For this review, use the dimensioned drawing (mm, ordinates from the lowest corner) and the shaded views. A direction names the side the tool comes from. Round coordinates to 2 decimals unless told otherwise and drop trailing zeros. Loops run counter-clockwise (first coordinate to the right, second up) from the corner with the lowest first, then second, coordinate; pieces in that order, holes last. Notation, with made-up numbers: (24.25, 84.5) -> (52.25, 84.5) arc R38 cw to (52.25, 123.5) -> close; hole circle Ø4 at (51, 89). An arc over 180 degrees is marked (long way). Write each question's results on one line, items separated by ' | '.
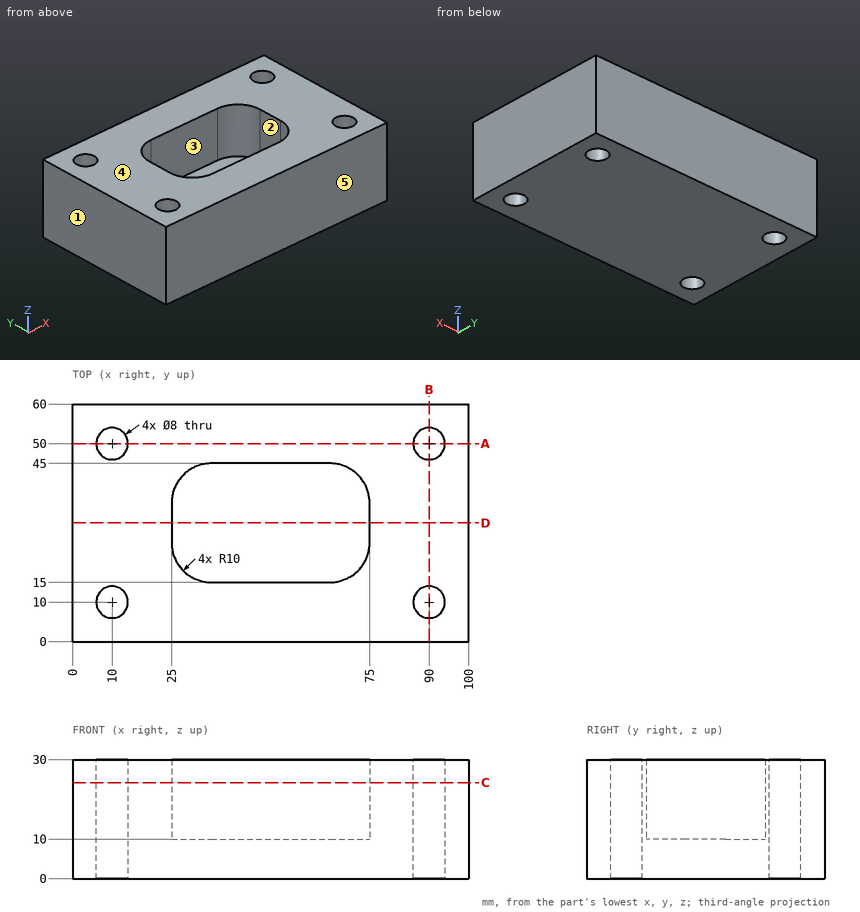
1. Draft analysis for pull direction Y (two halves, no side actions). For the marked faces 3, 4 and 5, state which applies: released by +Y, released by -Y, zero draft, split by the parting line, or undercut.
Values found:
face 3: undercut | face 4: zero draft | face 5: released by -Y
2. For pin 1 (5 mm diameter, centred on x = 10, y = 10, fed in from -Z); pin 2 (5 mm diameter, centred on x = 41, y = 22.5, fed in from +Z), all flat-tipped, find the tip position at first contact; note any pin that passes through.
Values found:
pin 1: passes through | pin 2: stops at z = 10
3. To check wall thickness, follow probe 1 along Y at (x, z) = (90, 19.25); probe 2 along Y at (x, z) = (57, 24); probe 3 along X at (y, z) = (50.5, 16.75). State the ranges of each line that lie inside material, in increasing order.
Values found:
probe 1: y = 0 to 6, 14 to 46, 54 to 60 | probe 2: y = 0 to 15, 45 to 60 | probe 3: x = 0 to 6.03, 13.97 to 86.03, 93.97 to 100
4. Consider section A-A (y = 50). State the section outline as (x, z) points.
Values found:
outline: (0, 0) -> (6, 0) -> (6, 30) -> (0, 30) -> close; (14, 0) -> (86, 0) -> (86, 30) -> (14, 30) -> close; (94, 0) -> (100, 0) -> (100, 30) -> (94, 30) -> close
5. Consider section D-D (y = 30). State the section outline as (x, z) points.
Values found:
outline: (0, 0) -> (100, 0) -> (100, 30) -> (75, 30) -> (75, 10) -> (25, 10) -> (25, 30) -> (0, 30) -> close
6. Consider section B-B (x = 90). State the section outline as (y, z) points, plus the area to 3 significant figures.
Values found:
outline: (0, 0) -> (6, 0) -> (6, 30) -> (0, 30) -> close; (14, 0) -> (46, 0) -> (46, 30) -> (14, 30) -> close; (54, 0) -> (60, 0) -> (60, 30) -> (54, 30) -> close | area: 1,320 mm2
7. Tool access review of the marked faces 1 and 2: name each direction out of +Z, -Z, +X, -X, +Y, -Y from which nothing blocks a thin tool from reaching the whole face with its end or side.
Values found:
face 1: +Z, -Z, -X, +Y, -Y | face 2: +Z
8. Consider section C-C (z = 24.25). State the section outline as (x, y) points, plus the area to 3 significant figures.
Values found:
outline: (0, 0) -> (100, 0) -> (100, 60) -> (0, 60) -> close; hole circle Ø8 at (10, 10); hole circle Ø8 at (10, 50); hole (25, 25) arc R10 ccw to (35, 15) -> (65, 15) arc R10 ccw to (75, 25) -> (75, 35) arc R10 ccw to (65, 45) -> (35, 45) arc R10 ccw to (25, 35) -> close; hole circle Ø8 at (90, 10); hole circle Ø8 at (90, 50) | area: 4,380 mm2
